Autodesk Inventor part; units mm, degrees
ref_plane "YZ Plane" through (0, 0, 0) normal (1, 0, 0) x (0, 1, 0)
ref_plane "XZ Plane" through (0, 0, 0) normal (0, 1, 0) x (-1, 0, 0)
ref_plane "XY Plane" through (0, 0, 0) normal (0, 0, 1) x (1, 0, 0)
sketch "Esquisse1" plane through (0, 0, 0) normal (0, 1, 0) x (-1, 0, 0)
  line L0 (0, 0) -> (110, 0)
  line L1 (110, 0) -> (110, -170)
  line L2 (110, -170) -> (0, -170)
  line L3 (0, -170) -> (0, 0)
  dimension "d0" = 110
  dimension "d1" = 170
extrude "Extrusion1" add sketch "Esquisse1" along normal blind 5
sketch "Esquisse2" plane through (0, 5, 0) normal (0, 1, 0) x (1, 0, 0)
  line L0 (-110, 0) -> (0, 0)
  line L1 (-110, 0) -> (-110, 5)
  line L2 (-110, 170) -> (-110, 0)
  line L3 (-110, 5) -> (-105, 5)
  line L4 (-105, 5) -> (-106, 5)
  line L5 (-106, 5) -> (-106, 20)
  line L6 (-106, 20) -> (-109, 20)
  line L7 (-109, 20) -> (-109, 5)
  line L8 (-55, 0) -> (-55, 170)
  line L9 (-55, 85) -> (-68.7933, 85)
  line L10 (0, 5) -> (-5, 5)
  line L11 (-4, 5) -> (-4, 20)
  line L12 (-4, 20) -> (-1, 20)
  line L13 (-1, 20) -> (-1, 5)
  line L14 (-110, 165) -> (-105, 165)
  line L15 (-106, 165) -> (-106, 150)
  line L16 (-106, 150) -> (-109, 150)
  line L17 (-109, 150) -> (-109, 165)
  line L18 (-4, 165) -> (-4, 150)
  line L19 (-1, 150) -> (-1, 165)
  line L20 (0, 165) -> (-5, 165)
  line L21 (-4, 150) -> (-1, 150)
  dimension "d4" = 5
  dimension "d5" = 5
  dimension "d6" = 1
  dimension "d7" = 15
  dimension "d8" = 3
  dimension "d9" = 90
  dimension "d10" = 13.7933
  dimension "d11" = 85
extrude "Extrusion2" cut sketch "Esquisse2" against normal blind 5
sketch "Esquisse3" plane through (0, 5, 0) normal (0, 1, 0) x (1, 0, 0)
  line L0 (-110, 0) -> (0, 0)
  line L1 (-110, 0) -> (-110, 70)
  line L2 (-110, 170) -> (-110, 0)
  line L3 (-110, 70) -> (-92.5, 70)
  line L4 (-92.5, 70) -> (-92.5, 85)
  line L5 (-92.5, 85) -> (-62.5, 85)
  line L6 (-62.5, 85) -> (-62.5, 70)
  dimension "d14" = 70
  dimension "d15" = 17.5
  dimension "d16" = 15
  dimension "d17" = 30
hole "Perçage1" at (-92.5, 5, -70) at (-92.5, 5, -85) at (-62.5, 5, -85) at (-62.5, 5, -70) direction (0, -1, 0) diameter 2.459 end through all
properties part number "châssis haut avant"
Can you work these out from the model? Positions are in its coordinate system, mm. A direction names the side the tool comes from. Round coordinates to 2 decimals unless told otherwise and drop trailing zeros. Use one line per item in the form item = value. Start each with the question number.
Q1. If I drill on probe 1 along Z at (x, y) = (-92.5, 2.4); probe 2 along X at (y, z) = (0.55, -12.5); probe 3 along X at (y, z) = (3.15, -70), over which ranges is the centre line in solid material (lowest first)? Write a range as [from, to].
Q2. We'd pull the mould along X, two halves only. Please class faces 1 (the face through (0, 2, -86)), 2 (the face through (-4, 3, -12)), 3 (the face through (-109, 3, -13)), 4 (the face through (-54, 0, -84)): +X half, -X half, draft (parallel to the pull), parting line (faces both ways), or undercut.
Q3. I'm going to push a flat-ended pin straight in: P1, Ø1.5, axis at x = -108, y = 1.5, coming from the +Z side. Where does the tip first touch, or does it pass through?
Q4. Which directions (+Z, -Z, +X, -X, +Y, -Y) give clear straight access to the entire face, cutting with the end or side of a thin tool? Please do faces 5 (the face through (-54, 5, -84)), 6 (the face through (-109, 3, -157)).
Worked out:
q1.probe_1 = [-170, -86.23], [-83.77, -71.23], [-68.77, 0]
q1.probe_2 = [-110, -109], [-106, -4], [-1, 0]
q1.probe_3 = [-110, -93.73], [-91.27, -63.73], [-61.27, 0]
q2.face_1 = +X half
q2.face_2 = undercut
q2.face_3 = undercut
q2.face_4 = draft
q3.P1 = 0
q4.face_5 = +Z, -Z, +X, -X, +Y
q4.face_6 = +Y, -Y
